from build123d import *

# Parameters (mm, degrees)
SKETCH5_R           = 1.5875
BOSS_EXTRUDE1_DEPTH = 3


with BuildPart() as part:
    # Sketch5 → Boss-Extrude1 (new body)
    with BuildSketch(Plane(origin=(0, 0, 0), x_dir=(1, 0, 0), z_dir=(0, 1, 0))):
        with BuildLine():
            Line((-3.25, -7), (83.25, -7))
            ThreePointArc((83.25, -7), (85.371320344, -6.121320344), (86.25, -4))
            Line((86.25, -4), (86.25, 54))
            ThreePointArc((86.25, 54), (85.371320344, 56.121320344), (83.25, 57))
            Line((83.25, 57), (-3.25, 57))
            ThreePointArc((-3.25, 57), (-5.371320344, 56.121320344), (-6.25, 54))
            Line((-6.25, 54), (-6.25, -4))
            ThreePointArc((-6.25, -4), (-5.371320344, -6.121320344), (-3.25, -7))
        make_face()
        with Locations(Location((2, 2, 0), (0, 0, 270))):
            Circle(SKETCH5_R, mode=Mode.SUBTRACT)
        with Locations(Location((2, 48, 0), (0, 0, 270))):
            Circle(SKETCH5_R, mode=Mode.SUBTRACT)
        with Locations(Location((78, 48, 0), (0, 0, 270))):
            Circle(SKETCH5_R, mode=Mode.SUBTRACT)
        with Locations(Location((78, 2, 0), (0, 0, 270))):
            Circle(SKETCH5_R, mode=Mode.SUBTRACT)
        with BuildLine():
            Line((10.353326987, 54), (21.153326987, 54))
            ThreePointArc((21.153326987, 54), (22.006880378, 54.353553391), (21.653326987, 53.5))
            Line((21.653326987, 53.5), (21.653326987, 51.5))
            ThreePointArc((21.653326987, 51.5), (22.006880378, 50.646446609), (21.153326987, 51))
            Line((21.153326987, 51), (10.353326987, 51))
            ThreePointArc((10.353326987, 51), (9.499773597, 50.646446609), (9.853326987, 51.5))
            Line((9.853326987, 51.5), (9.853326987, 53.5))
            ThreePointArc((9.853326987, 53.5), (9.499773597, 54.353553391), (10.353326987, 54))
        make_face(mode=Mode.SUBTRACT)
        with BuildLine():
            Line((58.85, 54), (69.65, 54))
            ThreePointArc((69.65, 54), (70.503553391, 54.353553391), (70.15, 53.5))
            Line((70.15, 53.5), (70.15, 51.5))
            ThreePointArc((70.15, 51.5), (70.503553391, 50.646446609), (69.65, 51))
            Line((69.65, 51), (58.85, 51))
            ThreePointArc((58.85, 51), (57.996446609, 50.646446609), (58.35, 51.5))
            Line((58.35, 51.5), (58.35, 53.5))
            ThreePointArc((58.35, 53.5), (57.996446609, 54.353553391), (58.85, 54))
        make_face(mode=Mode.SUBTRACT)
        with BuildLine():
            Line((10.35, -1), (21.15, -1))
            ThreePointArc((21.15, -1), (22.003553391, -0.646446609), (21.65, -1.5))
            Line((21.65, -1.5), (21.65, -3.5))
            ThreePointArc((21.65, -3.5), (22.003553391, -4.353553391), (21.15, -4))
            Line((21.15, -4), (10.35, -4))
            ThreePointArc((10.35, -4), (9.496446609, -4.353553391), (9.85, -3.5))
            Line((9.85, -3.5), (9.85, -1.5))
            ThreePointArc((9.85, -1.5), (9.496446609, -0.646446609), (10.35, -1))
        make_face(mode=Mode.SUBTRACT)
        with BuildLine():
            Line((58.85, -1), (69.65, -1))
            ThreePointArc((69.65, -1), (70.503553391, -0.646446609), (70.15, -1.5))
            Line((70.15, -1.5), (70.15, -3.5))
            ThreePointArc((70.15, -3.5), (70.503553391, -4.353553391), (69.65, -4))
            Line((69.65, -4), (58.85, -4))
            ThreePointArc((58.85, -4), (57.996446609, -4.353553391), (58.35, -3.5))
            Line((58.35, -3.5), (58.35, -1.5))
            ThreePointArc((58.35, -1.5), (57.996446609, -0.646446609), (58.85, -1))
        make_face(mode=Mode.SUBTRACT)
        with BuildLine():
            Line((-3.25, 9.6), (-3.25, 20.4))
            ThreePointArc((-3.25, 20.4), (-3.603553391, 21.253553391), (-2.75, 20.9))
            Line((-2.75, 20.9), (-0.75, 20.9))
            ThreePointArc((-0.75, 20.9), (0.103553391, 21.253553391), (-0.25, 20.4))
            Line((-0.25, 20.4), (-0.25, 9.6))
            ThreePointArc((-0.25, 9.6), (0.103553391, 8.746446609), (-0.75, 9.1))
            Line((-0.75, 9.1), (-2.75, 9.1))
            ThreePointArc((-2.75, 9.1), (-3.603553391, 8.746446609), (-3.25, 9.6))
        make_face(mode=Mode.SUBTRACT)
        with BuildLine():
            Line((-3.25, 29.6), (-3.25, 40.4))
            ThreePointArc((-3.25, 40.4), (-3.603553391, 41.253553391), (-2.75, 40.9))
            Line((-2.75, 40.9), (-0.75, 40.9))
            ThreePointArc((-0.75, 40.9), (0.103553391, 41.253553391), (-0.25, 40.4))
            Line((-0.25, 40.4), (-0.25, 29.6))
            ThreePointArc((-0.25, 29.6), (0.103553391, 28.746446609), (-0.75, 29.1))
            Line((-0.75, 29.1), (-2.75, 29.1))
            ThreePointArc((-2.75, 29.1), (-3.603553391, 28.746446609), (-3.25, 29.6))
        make_face(mode=Mode.SUBTRACT)
        with BuildLine():
            Line((80.25, 9.6), (80.25, 20.4))
            ThreePointArc((80.25, 20.4), (79.896446609, 21.253553391), (80.75, 20.9))
            Line((80.75, 20.9), (82.75, 20.9))
            ThreePointArc((82.75, 20.9), (83.603553391, 21.253553391), (83.25, 20.4))
            Line((83.25, 20.4), (83.25, 9.6))
            ThreePointArc((83.25, 9.6), (83.603553391, 8.746446609), (82.75, 9.1))
            Line((82.75, 9.1), (80.75, 9.1))
            ThreePointArc((80.75, 9.1), (79.896446609, 8.746446609), (80.25, 9.6))
        make_face(mode=Mode.SUBTRACT)
        with BuildLine():
            Line((80.25, 29.6), (80.25, 40.4))
            ThreePointArc((80.25, 40.4), (79.896446609, 41.253553391), (80.75, 40.9))
            Line((80.75, 40.9), (82.75, 40.9))
            ThreePointArc((82.75, 40.9), (83.603553391, 41.253553391), (83.25, 40.4))
            Line((83.25, 40.4), (83.25, 29.6))
            ThreePointArc((83.25, 29.6), (83.603553391, 28.746446609), (82.75, 29.1))
            Line((82.75, 29.1), (80.75, 29.1))
            ThreePointArc((80.75, 29.1), (79.896446609, 28.746446609), (80.25, 29.6))
        make_face(mode=Mode.SUBTRACT)
    extrude(amount=BOSS_EXTRUDE1_DEPTH)


solid = part.part
Geometry: final body of the model. Coordinates: model frame, mm. Round coordinates to 2 decimals unless told otherwise and drop trailing zeros. Loops run counter-clockwise (first coordinate to the right, second up) from the corner with the lowest first, then second, coordinate; pieces in that order, holes last. Notation, with made-up numbers: M 42.25,18 L 68.25,18 A25 ccw 68.25,51 Z; hole C 24.5,20 d9. An arc over 180 degrees is marked long. Put each result on its own line as item: value. Start each with the question number.
(1) Draft query along Z for faces 1 (the face through (41, 1, -57)), 2 (the face through (85.35, 1.48, 6.14)), 3 (the face through (64, 1, 4)), 4 (the face through (58.35, 1, 3)). Return one class per face: +Z half, -Z half, draft (parallel to the pull), parting line (faces both ways), or undercut.
(2) Section query C-C (y = 1.1). State how many separate pieces and enclosed holes the cut face has, then the cut area to 3 significant figures.
(3) Section query B-B (z = -38.5). Return loops of the section in (x, y).
(4) Section query A-A (x = 2). Return loops of the section in (y, z).
(5) Material intervals for line 1 along Z through (x, y) = (81, 2.75); line 2 along Z through (x, y) = (17, 1.1); line 3 along X through (y, z) = (1.55, -15.5), sorted ascending. Write a range as [from, to].
Findings below:
1. face 1: -Z half
1. face 2: +Z half
1. face 3: undercut
1. face 4: undercut
2. separate pieces: 1
2. enclosed holes: 12
2. area: 5,580 mm2
3. outline: M -6.25,0 L -3.25,0 L -3.25,3 L -6.25,3 Z; M -0.25,0 L 80.25,0 L 80.25,3 L -0.25,3 Z; M 83.25,0 L 86.25,0 L 86.25,3 L 83.25,3 Z
4. outline: M 0,-57 L 3,-57 L 3,-49.59 L 0,-49.59 Z; M 0,-46.41 L 3,-46.41 L 3,-3.59 L 0,-3.59 Z; M 0,-0.41 L 3,-0.41 L 3,7 L 0,7 Z
5. line 1: z = [-57, -40.9], [-29.1, -20.9], [-9.1, 7]
5. line 2: z = [-57, -54], [-51, 1], [4, 7]
5. line 3: x = [-6.25, -3.25], [-0.25, 80.25], [83.25, 86.25]
